Source: CAD feature listing. Evaluate the final solid. Frame: model axes, mm. A direction names the side the tool comes from. Coordinates: 2 decimals unless noted, no trailing zeros. Loops run counter-clockwise (first coordinate to the right, second up) from the corner with the lowest first, then second, coordinate; pieces in that order, holes last.
from build123d import *

# Parameters (mm, degrees)
SKETCH1_W           = 55
SKETCH1_H           = 54
MAINSHAPE_DEPTH     = 4.5
SKETCH2_W           = 10
SKETCH2_H           = 9
TAB1_DEPTH          = 4.5
CUT_EXTRUDE2_DEPTH  = 43.056509603
SKETCH5_W           = 4.7
SKETCH5_H           = 10.2
CUT_EXTRUDE3_DEPTH  = 43.056509603
SKETCH6_R           = 12
CUT_EXTRUDE4_DEPTH  = 43.056509603
SKETCH8_R           = 1.55
CUT_EXTRUDE6_DEPTH  = 43.056509603
SKETCH11_R          = 1.55
CUT_EXTRUDE8_DEPTH  = 43.056509603
SKETCH15_R          = 12
SKETCH15_R_2        = 6
BOSS_EXTRUDE2_DEPTH = 4.5
CUT_EXTRUDE10_DEPTH = 43.056509603


with BuildPart() as part:
    # Sketch1 → MainShape (new body)
    with BuildSketch(Plane(origin=(0, 0, 0), x_dir=(1, 0, 0), z_dir=(0, 1, 0))):
        Rectangle(SKETCH1_W, SKETCH1_H)
    extrude(amount=MAINSHAPE_DEPTH)

    # Sketch2 → Tab1 (add, through all)
    with BuildSketch(Plane(origin=(0, 4.5, 0), x_dir=(1, 0, 0), z_dir=(0, 1, 0))):
        with Locations((0, 27)):
            Rectangle(SKETCH2_W, SKETCH2_H)
    extrude(amount=-TAB1_DEPTH)

    # Sketch4 → Cut-Extrude2 (cut, through all)
    with BuildSketch(Plane(origin=(0, 4.5, 0), x_dir=(1, 0, 0), z_dir=(0, 1, 0))):
        with BuildLine():
            Line((-13.25, 16.5), (-16.75, 16.5))
            Line((-16.75, 16.5), (-16.75, 19))
            Line((-16.75, 19), (-17.75, 19))
            ThreePointArc((-17.75, 19), (-17.926776695, 19.073223305), (-18, 19.25))
            Line((-18, 19.25), (-18, 22.95))
            ThreePointArc((-18, 22.95), (-17.926776695, 23.126776695), (-17.75, 23.2))
            Line((-17.75, 23.2), (-16.75, 23.2))
            Line((-16.75, 23.2), (-16.75, 27))
            Line((-16.75, 27), (-13.25, 27))
            Line((-13.25, 27), (-13.25, 23.2))
            Line((-13.25, 23.2), (-12.25, 23.2))
            ThreePointArc((-12.25, 23.2), (-12.073223305, 23.126776695), (-12, 22.95))
            Line((-12, 22.95), (-12, 19.25))
            ThreePointArc((-12, 19.25), (-12.073223305, 19.073223305), (-12.25, 19))
            Line((-12.25, 19), (-13.25, 19))
            Line((-13.25, 19), (-13.25, 16.5))
        make_face()
        with BuildLine():
            Line((13.25, 16.5), (13.25, 19))
            Line((13.25, 19), (12.25, 19))
            ThreePointArc((12.25, 19), (12.073223305, 19.073223305), (12, 19.25))
            Line((12, 19.25), (12, 22.95))
            ThreePointArc((12, 22.95), (12.073223305, 23.126776695), (12.25, 23.2))
            Line((12.25, 23.2), (13.25, 23.2))
            Line((13.25, 23.2), (13.25, 27))
            Line((13.25, 27), (16.75, 27))
            Line((16.75, 27), (16.75, 23.2))
            Line((16.75, 23.2), (17.75, 23.2))
            ThreePointArc((17.75, 23.2), (17.926776695, 23.126776695), (18, 22.95))
            Line((18, 22.95), (18, 19.25))
            ThreePointArc((18, 19.25), (17.926776695, 19.073223305), (17.75, 19))
            Line((17.75, 19), (16.75, 19))
            Line((16.75, 19), (16.75, 16.5))
            Line((16.75, 16.5), (13.25, 16.5))
        make_face()
    extrude(amount=-CUT_EXTRUDE2_DEPTH, mode=Mode.SUBTRACT)

    # Sketch5 → Cut-Extrude3 (cut, through all)
    with BuildSketch(Plane(origin=(0, 4.5, 0), x_dir=(1, 0, 0), z_dir=(0, 1, 0))):
        with Locations((23, 7)):
            Rectangle(SKETCH5_W, SKETCH5_H)
        with Locations((-23, 7)):
            Rectangle(SKETCH5_W, SKETCH5_H)
        with Locations((-23, -13)):
            Rectangle(SKETCH5_W, SKETCH5_H)
        with Locations((23, -13)):
            Rectangle(SKETCH5_W, SKETCH5_H)
    extrude(amount=-CUT_EXTRUDE3_DEPTH, mode=Mode.SUBTRACT)

    # Sketch6 → Cut-Extrude4 (cut, through all)
    with BuildSketch(Plane(origin=(0, 4.5, 0), x_dir=(1, 0, 0), z_dir=(0, 1, 0))):
        with Locations(Location((0, 1, 0), (0, 0, 270))):
            Circle(SKETCH6_R)
    extrude(amount=-CUT_EXTRUDE4_DEPTH, mode=Mode.SUBTRACT)

    # Sketch8 → Cut-Extrude6 (cut, through all)
    with BuildSketch(Plane(origin=(0, 4.5, 0), x_dir=(1, 0, 0), z_dir=(0, 1, 0))):
        with Locations(Location((-8, -20.46, 0), (0, 0, 270))):
            Circle(SKETCH8_R)
        with Locations(Location((8, -20.46, 0), (0, 0, 90))):
            Circle(SKETCH8_R)
    extrude(amount=-CUT_EXTRUDE6_DEPTH, mode=Mode.SUBTRACT)

    # Sketch11 → Cut-Extrude8 (cut, through all)
    with BuildSketch(Plane(origin=(0, 4.5, 0), x_dir=(1, 0, 0), z_dir=(0, 1, 0))):
        with Locations(Location((-23, 19.5, 0), (0, 0, 270))):
            Circle(SKETCH11_R)
        with Locations(Location((23, 19.5, 0), (0, 0, 90))):
            Circle(SKETCH11_R)
    extrude(amount=-CUT_EXTRUDE8_DEPTH, mode=Mode.SUBTRACT)

    # Sketch15 → Boss-Extrude2 (add, through all)
    with BuildSketch(Plane(origin=(0, 4.5, 0), x_dir=(1, 0, 0), z_dir=(0, 1, 0))):
        with Locations((0, 1)):
            Circle(SKETCH15_R)
        with Locations(Location((0, 1, 0), (0, 0, 270))):
            Circle(SKETCH15_R_2, mode=Mode.SUBTRACT)
    extrude(amount=-BOSS_EXTRUDE2_DEPTH)

    # Sketch16 → Cut-Extrude10 (cut, through all)
    with BuildSketch(Plane(origin=(0, 4.5, 0), x_dir=(1, 0, 0), z_dir=(0, 1, 0))):
        with BuildLine():
            Line((0, 7), (2.479202711, 7))
            ThreePointArc((2.479202711, 7), (17, 1), (2.479202711, -5))
            Line((2.479202711, -5), (0, -5))
            Line((0, -5), (0, 7))
        make_face()
    extrude(amount=-CUT_EXTRUDE10_DEPTH, mode=Mode.SUBTRACT)


solid = part.part
Q1. Section C-C, the plane z = -1. Return the cut outline in (x, y).
Q2. Section B-B, the plane x = -8. Return the cut outline in (y, z), plus the area to 3 significant figures.
Q3. Contact query for a flat-ended pin moving along its axis: pin 1 Ø1.1 at (x, y) = (-12.5, 2.5) entering from -Z. Output: stop coordinate, or through.
Q4. Line query: line 1 along Z through (x, y) = (8, 2.95); line 2 along X through (y, z) = (3.6, -21.5); line 3 along X through (y, z) = (3.6, 20.5). Output: solid intervals per line, ascending.
Q5. Draft query along Z for faces 1 (the flat face through (-15, 2, -16.5)), 2 (the flat face through (23, 2, 18.1)), 3 (the flat face through (13.25, 2, -18)). Return one class per face: +Z half, -Z half, draft (parallel to the pull), parting line (faces both ways), or undercut.
Q6. Section A-A, the plane z = 14. Return the cut outline in (x, y), plus the area to 3 significant figures.
Q7. Section D-D, the plane z = -20. Return the cut outline in (x, y).
Q8. Access query for faces 4 (the flat face through (16.75, 2, -25)), 5 (the cylindrical face through (-6, 2, -1)), 6 (the flat face through (9, 2, -27)), 7 (the flat face through (-5, 2, -29)). Directions: +Z, -Z, +X, -X, +Y, -Y. A direction counts if a zero-diameter tool reaches every point of the face in a straight line with its end or side. Return the directions, or none.
Derived:
1. outline: (-27.5, 0) - (-6, 0) - (-6, 4.5) - (-27.5, 4.5) - close; (17, 0) - (27.5, 0) - (27.5, 4.5) - (17, 4.5) - close
2. outline: (0, -27) - (4.5, -27) - (4.5, 18.91) - (0, 18.91) - close; (0, 22.01) - (4.5, 22.01) - (4.5, 27) - (0, 27) - close
2. area: 229 mm2
3. pin 1: stops at z = -27
4. line 1: z = -27 to -9.49, 7.49 to 18.91, 22.01 to 27
4. line 2: x = -27.5 to -18, -12 to 12, 18 to 27.5
4. line 3: x = -27.5 to -9.55, -6.45 to 6.45, 9.55 to 27.5
5. face 1: -Z half
5. face 2: undercut
5. face 3: draft
6. outline: (-27.5, 0) - (-25.35, 0) - (-25.35, 4.5) - (-27.5, 4.5) - close; (-20.65, 0) - (20.65, 0) - (20.65, 4.5) - (-20.65, 4.5) - close; (25.35, 0) - (27.5, 0) - (27.5, 4.5) - (25.35, 4.5) - close
6. area: 205 mm2
7. outline: (-27.5, 0) - (-24.47, 0) - (-24.47, 4.5) - (-27.5, 4.5) - close; (-21.53, 0) - (-18, 0) - (-18, 4.5) - (-21.53, 4.5) - close; (-12, 0) - (12, 0) - (12, 4.5) - (-12, 4.5) - close; (18, 0) - (21.53, 0) - (21.53, 4.5) - (18, 4.5) - close; (24.47, 0) - (27.5, 0) - (27.5, 4.5) - (24.47, 4.5) - close
8. face 4: -Z, +Y, -Y
8. face 5: +Y, -Y
8. face 6: -Z, +X, +Y, -Y
8. face 7: -Z, -X, +Y, -Y
